```python
from build123d import *

# Parameters (mm, degrees)
SKETCH3_W          = 68
SKETCH3_H          = 68
CUT_EXTRUDE1_DEPTH = 4


with BuildPart() as part:
    # Sketch1 → Revolve1 (revolve)
    with BuildSketch(Plane.XY):
        Polygon((0, 23), (7, 23), (8.4, 22.624871131), (8.4, 19.375128869), (7, 19), (0, 19), align=None)
    revolve(axis=Axis((0, 19, 0), (0, 1, 0)))

    # Sketch2 → Cut-Revolve1 (revolve, cut)
    with BuildSketch(Plane.XY):
        Polygon((0, 23), (6, 23), (5.4585, 22.4585), (5.4585, 19.5415), (6, 19), (0, 19), align=None)
    revolve(axis=Axis((0, 19, 0), (0, 1, 0)), mode=Mode.SUBTRACT)

    # Sketch3 → Cut-Extrude1 (cut)
    with BuildSketch(Plane(origin=(0, 19, 0), x_dir=(-1, 0, 0), z_dir=(0, 1, 0))):
        Rectangle(SKETCH3_W, SKETCH3_H)
        Polygon((8.082903769, 0), (4.041451884, 7), (-4.041451884, 7), (-8.082903769, 0), (-4.041451884, -7), (4.041451884, -7), align=None, mode=Mode.SUBTRACT)
    extrude(amount=CUT_EXTRUDE1_DEPTH, mode=Mode.SUBTRACT)


solid = part.part
```
Geometry check sheet. Reference: the model listing, model coordinates, mm. Round coordinates to 2 decimals unless told otherwise and drop trailing zeros. Order: outer loops, then holes, each group sorted by start corner. A loop starts at its lowest first (then second) coordinate and runs counter-clockwise, first axis right, second up. Notation, with made-up numbers: (70, -40) - (100, -40) arc R29 cw to (100, -19) - close; hole circle Ø8 at (-38, 56). An arc over 180 degrees is marked (long way). Use a Markdown table: item, result. Add a question column.
1) Section check A-A (y = 22). Record the cut outline in (x, z).
2) Gauge pin test, flat ends, axial feed: P1, Ø8, axis at x = 2, z = 4, coming from the +Y side; P2, Ø1.5, axis at y = 21.5, z = 1, coming from the +X side. Record the tip position at first contact, or that the pin passes through.
3) Thickness scan on line 1 along X through (y, z) = (19.8, 0.75); line 2 along Z through (x, y) = (0.75, 20.3); line 3 along Z through (x, y) = (1.5, 21.5). Record the ranges inside material, lowest first.
Established:
| question | item | result |
|---|---|---|
| 1 | outline | (-8.08, 0) - (-4.04, -7) - (4.04, -7) - (8.08, 0) - (4.04, 7) - (-4.04, 7) - close; hole circle Ø10.92 at (0, 0) |
| 2 | P1 | y = 23 |
| 2 | P2 | x = 7.94 |
| 3 | line 1 | -7.65 to -5.41, 5.41 to 7.65 |
| 3 | line 2 | -7 to -5.41, 5.41 to 7 |
| 3 | line 3 | -7 to -5.25, 5.25 to 7 |
